Design review of the part built by this model. Coordinates are the model's own, in mm. A direction names the side the tool comes from. Coordinates: 2 decimals unless noted, no trailing zeros. Order: outer loops, then holes, each group sorted by start corner. A loop starts at its lowest first (then second) coordinate and runs counter-clockwise, first axis right, second up. Notation, with made-up numbers: (79, -16.75) -> (90, -16.75) arc R20 ccw to (90, 22.25) -> close; hole circle Ø5 at (-39, -23). An arc over 180 degrees is marked (long way). Write item = value, one per line.
```python
from build123d import *

# Parameters (mm, degrees)
BOSS_EXTRUDE1_DEPTH = 16
BOSS_EXTRUDE2_START = -27
SKETCH3_R           = 7.5
BOSS_EXTRUDE2_DEPTH = 27
SKETCH7_W           = 15
SKETCH7_H           = 50
CUT_EXTRUDE1_DEPTH  = 63
SKETCH8_R           = 7.5
BOSS_EXTRUDE6_DEPTH = 12
SKETCH9_R           = 7.5
CUT_EXTRUDE2_DEPTH  = 26


with BuildPart() as part:
    # Sketch1 → Boss-Extrude1 (new body, symmetric)
    with BuildSketch(Plane(origin=(0, 0, 0), x_dir=(1, 0, 0), z_dir=(0, 1, 0))):
        with BuildLine():
            Line((0, 13), (0, 25))
            ThreePointArc((0, 25), (-25, 0), (0, -25))
            Line((0, -25), (0, -13))
            ThreePointArc((0, -13), (-13, 0), (0, 13))
        make_face()
    extrude(amount=BOSS_EXTRUDE1_DEPTH, both=True)

    # Sketch3 → Boss-Extrude2 (add)
    with BuildSketch(Plane.XY.offset(40).offset(BOSS_EXTRUDE2_START)):
        with BuildLine():
            Line((0, 16), (0, -16))
            ThreePointArc((0, -16), (10.310830972, -13.799251334), (19.882176961, -18.220322017))
            ThreePointArc((19.882176961, -18.220322017), (62, 0), (19.882176961, 18.220322017))
            ThreePointArc((19.882176961, 18.220322017), (10.310830972, 13.799251334), (0, 16))
        make_face()
        with Locations((37, 0)):
            Circle(SKETCH3_R, mode=Mode.SUBTRACT)
    extrude(amount=BOSS_EXTRUDE2_DEPTH)

    # Sketch7 → Cut-Extrude1 (cut, through all)
    with BuildSketch(Plane.ZY):
        with Locations((32.5, 0)):
            Rectangle(SKETCH7_W, SKETCH7_H)
    extrude(amount=-CUT_EXTRUDE1_DEPTH, mode=Mode.SUBTRACT)

    # Sketch8 → Boss-Extrude6 (add)
    with BuildSketch(Plane.XY.offset(-25)):
        with BuildLine():
            Line((0, -16), (0, 16))
            ThreePointArc((0, 16), (10.310830972, 13.799251334), (19.882176961, 18.220322017))
            ThreePointArc((19.882176961, 18.220322017), (62, 0), (19.882176961, -18.220322017))
            ThreePointArc((19.882176961, -18.220322017), (10.310830972, -13.799251334), (0, -16))
        make_face()
        with Locations((37, 0)):
            Circle(SKETCH8_R, mode=Mode.SUBTRACT)
    extrude(amount=BOSS_EXTRUDE6_DEPTH)

    # Sketch9 → Cut-Extrude2 (cut, through all)
    with BuildSketch(Plane(origin=(0, 0, 0), x_dir=(0, 0, -1), z_dir=(1, 0, 0))):
        Circle(SKETCH9_R)
    extrude(amount=-CUT_EXTRUDE2_DEPTH, mode=Mode.SUBTRACT)


solid = part.part
```
(1) We need section D-D (y = -3.5). Write out the cut boundary in (x, z), and give its area (3 significant figures).
Report:
outline = (-24.1, -6.63) arc R25 ccw to (0, -25) -> (30.37, -25) -> (30.37, -13) -> (0, -13) arc R13 cw to (-11.18, -6.63) -> close; (-24.1, 6.63) -> (-11.18, 6.63) arc R13 cw to (0, 13) -> (30.37, 13) -> (30.37, 25) -> (0, 25) arc R25 ccw to start; (43.63, -25) -> (61.75, -25) -> (61.75, -13) -> (43.63, -13) -> close; (43.63, 13) -> (61.75, 13) -> (61.75, 25) -> (43.63, 25) -> close
area = 1,720 mm²
(2) The part is to be moulded in two halves that separate along Z. For faces 4 (the cylindrical face through (-9.772, 0.224, 8.573)), 5 (the flat face through (-15, 16, 0)), 6 (the flat face through (31, 6, 13)), 7 (the flat face through (31, -5, -25)), say which applies: released by +Z, released by -Z, zero draft, split by the parting line, or undercut.
Report:
face_4 = undercut
face_5 = zero draft
face_6 = undercut
face_7 = released by -Z
(3) For faces 1 (the flat face through (-15, -16, 0)), 2 (the flat face through (31, -5, -13)), 3 (the flat face through (31, -6, 25)), list the 3-axis set-ups (+Z, -Z, +X, -X, +Y, -Y) from which the entire face can be reached by the end or side of a thin tool; tool diameter is ignored.
Report:
face_1 = +Z, -Z, -X, -Y
face_2 = +X, +Y, -Y
face_3 = +Z, +X, -X, +Y, -Y
(4) We need section A-A (z = 0). Write out the cut boundary in (x, y).
Report:
outline = (-25, -16) -> (-13, -16) -> (-13, -7.5) -> (-25, -7.5) -> close; (-25, 7.5) -> (-13, 7.5) -> (-13, 16) -> (-25, 16) -> close
(5) Insertion check: pin 1 (9 mm diameter, centred on y = 0, z = 0, fed in from -X); pin 2 (1.5 mm diameter, centred on y = -10, z = -5, fed in from +X); pin 3 (24 mm diameter, centred on x = 37, y = 0, fed in from -Z); pin 4 (8 mm diameter, centred on y = 9.5, z = 14, fed in from +X). Each pin has a flat end and moves straight along its axis. Give the tip position at first contact, or say it passes through.
Report:
pin_1 = through
pin_2 = -11.66
pin_3 = -25
pin_4 = 61.39
(6) We need section B-B (z = 20). Write out the cut boundary in (x, y).
Report:
outline = (-15, -16) -> (0, -16) arc R16.68 cw to (19.88, -18.22) arc R25 ccw (long way) to (19.88, 18.22) arc R16.68 cw to (0, 16) -> (-15, 16) -> close; hole circle Ø15 at (37, 0)
(7) For L1, parallel to Y at x = 37, z = 17; L2, parallel to Z at x = 41.5, y = -9.5; L3, parallel to Y at x = -17.5, z = 0, list the stretches that pass through material, from the lowest coordinate up.
Report:
L1 = -25 to -7.5, 7.5 to 25
L2 = -25 to -13, 13 to 25
L3 = -16 to -7.5, 7.5 to 16
(8) We need section C-C (x = 8). Write out the cut boundary in (y, z).
Report:
outline = (-13.7, -25) -> (13.7, -25) -> (13.7, -13) -> (-13.7, -13) -> close; (-13.7, 13) -> (13.7, 13) -> (13.7, 25) -> (-13.7, 25) -> close
